```python
from build123d import *

# Parameters (mm, degrees)
F1_DEPTH = 48
F2_R     = 6.5
F3_DEPTH = 11
F5_W     = 13
F5_H     = 16
F6_DEPTH = 12


with BuildPart() as f1:
    # F0 (on Front) → F1 (new body)
    with BuildSketch(Plane.XZ):
        with BuildLine():
            ThreePointArc((-19, -5.5), (0, 19.78004), (19, -5.5))
            Line((19, -5.5), (53.5, -5.5))
            Line((53.5, -5.5), (53.5, 5.5))
            Line((53.5, 5.5), (53.5, 35.5))
            Line((53.5, 35.5), (42.5, 35.5))
            Line((42.5, 35.5), (42.5, 5.5))
            Line((42.5, 5.5), (29.491524, 5.5))
            ThreePointArc((29.491524, 5.5), (0, 30), (-29.491524, 5.5))
            Line((-29.491524, 5.5), (-53.5, 5.5))
            Line((-53.5, 5.5), (-53.5, -5.5))
            Line((-53.5, -5.5), (-19, -5.5))
        make_face()
    extrude(amount=F1_DEPTH)

    # F2 (on face) → F3 (cut)
    with BuildSketch(Plane.XY.offset(5.5)):
        with Locations((-41.495762, -35)):
            Circle(F2_R)
        with Locations((-41.495762, -13)):
            Circle(F2_R)
    extrude(amount=-F3_DEPTH, mode=Mode.SUBTRACT)

    # F5 (on face) → F6 (cut)
    with BuildSketch(Plane.YZ.offset(53.5)):
        with BuildLine():
            Line((-17.5, 19.5), (-30.5, 19.5))
            ThreePointArc((-30.5, 19.5), (-24, 13), (-17.5, 19.5))
        make_face()
        with Locations((-24, 27.5)):
            Rectangle(F5_W, F5_H)
    extrude(amount=-F6_DEPTH, mode=Mode.SUBTRACT)


solid = f1.part
```
Geometry: final body of the model. Coordinates: model frame, mm. A direction names the side the tool comes from. Round coordinates to 2 decimals unless told otherwise and drop trailing zeros. Order: outer loops, then holes, each group sorted by start corner. A loop starts at its lowest first (then second) coordinate and runs counter-clockwise, first axis right, second up. Notation, with made-up numbers: (4.25, 84.5) -> (10.25, 84.5) arc R31 cw to (10.25, 108.5) -> close; hole circle Ø5 at (-6.75, 71.5). An arc over 180 degrees is marked (long way). Use one line per item in the form item = value. Start each with the question number.
1. Cut plane D-D (y = -24). Return the cut outline in (x, z).
2. Cut plane B-B (y = -35). Return the cut outline in (x, z), then the cut area to 3 significant figures.
3. Pin query (flat end, axial travel): pin 1 Ø6.5 at (x, y) = (36.5, -26.5) entering from +Z; pin 2 Ø1.5 at (x, y) = (-11, -12.5) entering from -Z; pin 3 Ø5.5 at (x, z) = (50, 30.5) entering from +Y; pin 4 Ø15 at (y, z) = (-25.5, 20.5) entering from -X. Return the tip coordinate at first contact, or that it passes through.
4. Draft query along X for faces 6 (the face through (53.5, -24, 10)), 7 (the face through (-35.296, -11.048, 0.077)), 8 (the face through (-36, -24, -5.5)). Return one class per face: pulls with the +X half, pulls with the -X half, needs draft (parallel to the pull), parting line crosses it, or undercut.
5. Reachability of faces 1 (the face through (-0.513, -23.664, 19.773)), 2 (the face through (48, -9, 35.5)), 3 (the face through (48, -24, 13)), 4 (the face through (36, -24, 5.5)), 5 (the face through (-41, -24, 5.5)) from +Z, -Z, +X, -X, +Y, -Y: full face, straight path, thin tool, end or side. Return the list, or none.
6. Line query: probe 1 along Y at (x, z) = (-41, -3.5); probe 2 along X at (y, z) = (-19, 0); probe 3 along X at (y, z) = (-34, 3). Output: solid intervals per line, ascending.
7. Cut plane A-A (z = 0). Return the cut outline in (x, y), then the cut area to 3 significant figures.
8. Cut plane C-C (z = 32). Return the cut outline in (x, y), then the cut area to 3 significant figures.
Solution:
q1.outline = (-53.5, -5.5) -> (-19, -5.5) arc R19.78 cw (long way) to (19, -5.5) -> (53.5, -5.5) -> (53.5, 13) -> (42.5, 13) -> (42.5, 5.5) -> (29.49, 5.5) arc R30 ccw to (-29.49, 5.5) -> (-53.5, 5.5) -> close
q2.outline = (-53.5, -5.5) -> (-48, -5.5) -> (-48, 5.5) -> (-53.5, 5.5) -> close; (-35, -5.5) -> (-19, -5.5) arc R19.78 cw (long way) to (19, -5.5) -> (53.5, -5.5) -> (53.5, 35.5) -> (42.5, 35.5) -> (42.5, 5.5) -> (29.49, 5.5) arc R30 ccw to (-29.49, 5.5) -> (-35, 5.5) -> close
q2.area = 1,620 mm^2
q3.pin_1 = 5.5
q3.pin_2 = 15.91
q3.pin_3 = 0
q3.pin_4 = -27.04
q4.face_6 = pulls with the +X half
q4.face_7 = undercut
q4.face_8 = needs draft
q5.face_1 = +Y, -Y
q5.face_2 = +Z, +X, -X, +Y, -Y
q5.face_3 = +Z, +X
q5.face_4 = +Z, +Y, -Y
q5.face_5 = +Z, -X, +Y, -Y
q6.probe_1 = -48 to -41.48, -28.52 to -19.48, -6.52 to 0
q6.probe_2 = -53.5 to -44, -39 to -19.78, 19.78 to 53.5
q6.probe_3 = -53.5 to -47.92, -35.07 to -19.55, 19.55 to 53.5
q7.outline = (-53.5, -48) -> (-19.78, -48) -> (-19.78, 0) -> (-53.5, 0) -> close; (19.78, -48) -> (53.5, -48) -> (53.5, 0) -> (19.78, 0) -> close; hole circle Ø13 at (-41.5, -35); hole circle Ø13 at (-41.5, -13)
q7.area = 2,970 mm^2
q8.outline = (42.5, -48) -> (53.5, -48) -> (53.5, -30.5) -> (42.5, -30.5) -> close; (42.5, -17.5) -> (53.5, -17.5) -> (53.5, 0) -> (42.5, 0) -> close
q8.area = 385 mm^2
